Here's how the part is built. I have some questions about the finished solid (model axes, mm). A direction names the side the tool comes from. Round coordinates to 2 decimals unless told otherwise and drop trailing zeros. Order: outer loops, then holes, each group sorted by start corner. A loop starts at its lowest first (then second) coordinate and runs counter-clockwise, first axis right, second up. Notation, with made-up numbers: (22, 35.25) -> (79, 35.25) arc R8 cw to (79, 39.25) -> close; hole circle Ø5 at (-22, 35.25). An arc over 180 degrees is marked (long way). Use a Markdown table: item, result. Add a question column.
(1) I want a section at D-D, the plane z = 1. Give the number of separate pieces and of enclosed holes in the cut face, then the cut area to 3 significant figures.
(2) I want a section at A-A, the plane x = -1.5. Please give me the cut outline in (y, z).
(3) I want a section at C-C, the plane x = -8.5. Please give me the cut outline in (y, z).
(4) If I drill on probe 1 along Y at (x, z) = (0, 1); probe 2 along Y at (x, z) = (-3, 5.5); probe 3 along X at (y, z) = (-3.75, 0.5), over which ranges is the centre line in solid material (lowest first)?
(5) Thinking about a two-plate mould opening in X: for faces 4 (the face through (0, -7.05, 22)), 5 (the face through (-14.42, -4.03, 21.76)), 6 (the face through (6.9, 0, 2)), which applies, pulls with the +X half, pulls with the -X half, needs draft (parallel to the pull), parting line crosses it, or undercut?
(6) On a 3-axis mill with a long thin cutter (end or side, diameter ignored), from which of +Z, -Z, +X, -X, +Y, -Y can I reach the whole of each face in a straight line? I mean faces 1 (the face through (0, 2.8, -1)), 2 (the face through (-14.48, 3.97, 21.76)), 3 (the face through (-12.15, -2, 22)). Say none if no direction works.
(7) I'm going to push flat-ended pins straight in: P1, Ø6, axis at x = -0.5, y = 0, coming from the +Z side; P2, Ø1, axis at x = -13.5, z = 36.5, coming from the -Y side; P3, Ø0.6, axis at x = -13.5, z = 28, coming from the +Y side. Where does each tip first touch, or does it pass through?
from build123d import *

# Parameters (mm, degrees)
F1_DEPTH     = 2
F2_DEPTH     = 5
F3_DEPTH     = 44
F4_DEPTH     = 46.2
F6_T1_DEPTH  = 6.8
F6_T3_DEPTH  = 13.8
F6_T9_DEPTH  = 16.371682988
F6_T15_DEPTH = 9.371682988
F6_T24_DEPTH = 9.371682988
F6_T30_DEPTH = 16.371682988
F6_T39_DEPTH = 16.371682988
F6_T45_DEPTH = 9.371682988
F6_T54_DEPTH = 16.371682988
F6_T60_DEPTH = 9.371682988


# Not quite as in the source:
# - a fillet or chamfer that OpenCascade refuses, or shapes differently, is made with other operations: its cross-section is extruded or revolved along the edge and cut away or added
# - a feature names something its author has since deleted; it is built from what else it names


with BuildPart() as f1:
    # F0 (on Top) → F1 (new body)
    with BuildSketch(Plane.XY):
        with BuildLine():
            Line((10.3671572875, 5.05), (0, 5.05))
            Line((0, 5.05), (0, 4.2))
            Line((0, 4.2), (7.7, 4.2))
            Line((7.7, 4.2), (7.7, -4.2))
            Line((7.7, -4.2), (0, -4.2))
            Line((0, -4.2), (0, -5.05))
            Line((0, -5.05), (10.3671572875, -5.05))
            ThreePointArc((10.3671572875, -5.05), (10.5584990037, -5.0119397663), (10.7207106781, -4.9035533906))
            Line((10.7207106781, -4.9035533906), (12.15, -3.4742640687))
            Line((12.15, -3.4742640687), (12.15, -1.4742640687))
            Line((12.15, -1.4742640687), (14.15, -1.4742640687))
            Line((14.15, -1.4742640687), (15.2707106781, -0.3535533906))
            ThreePointArc((15.2707106781, -0.3535533906), (15.4171572875, 0), (15.2707106781, 0.3535533906))
            Line((15.2707106781, 0.3535533906), (10.7207106781, 4.9035533906))
            ThreePointArc((10.7207106781, 4.9035533906), (10.5584990037, 5.0119397663), (10.3671572875, 5.05))
        make_face()
        Polygon((6.9, 3.4), (0, 3.4), (0, 2.8), (6.3, 2.8), (6.3, -2.8), (0, -2.8), (0, -3.4), (6.9, -3.4), align=None)
        Polygon((7.7, 4.2), (0, 4.2), (0, 3.4), (6.9, 3.4), (6.9, -3.4), (0, -3.4), (0, -4.2), (7.7, -4.2), align=None)
        with BuildLine():
            Line((10.45, 7.05), (0, 7.05))
            Line((0, 7.05), (0, 5.85))
            Line((0, 5.85), (10.3671572875, 5.85))
            ThreePointArc((10.3671572875, 5.85), (10.8646457496, 5.7510433923), (11.2863961031, 5.4692388155))
            Line((11.2863961031, 5.4692388155), (15.8363961031, 0.9192388155))
            ThreePointArc((15.8363961031, 0.9192388155), (16.2171572875, 0), (15.8363961031, -0.9192388155))
            Line((15.8363961031, -0.9192388155), (11.2863961031, -5.4692388155))
            ThreePointArc((11.2863961031, -5.4692388155), (10.8646457496, -5.7510433923), (10.3671572875, -5.85))
            Line((10.3671572875, -5.85), (0, -5.85))
            Line((0, -5.85), (0, -7.05))
            Line((0, -7.05), (10.45, -7.05))
            ThreePointArc((10.45, -7.05), (11.3301718944, -6.8749229248), (12.0763455967, -6.3763455967))
            Line((12.0763455967, -6.3763455967), (16.8263455967, -1.6263455967))
            ThreePointArc((16.8263455967, -1.6263455967), (17.5, 0), (16.8263455967, 1.6263455967))
            Line((16.8263455967, 1.6263455967), (12.0763455967, 6.3763455967))
            ThreePointArc((12.0763455967, 6.3763455967), (11.3301718944, 6.8749229248), (10.45, 7.05))
        make_face()
        with BuildLine():
            Line((10.3671572875, 5.85), (0, 5.85))
            Line((0, 5.85), (0, 5.05))
            Line((0, 5.05), (10.3671572875, 5.05))
            ThreePointArc((10.3671572875, 5.05), (10.5584990037, 5.0119397663), (10.7207106781, 4.9035533906))
            Line((10.7207106781, 4.9035533906), (15.2707106781, 0.3535533906))
            ThreePointArc((15.2707106781, 0.3535533906), (15.4171572875, 0), (15.2707106781, -0.3535533906))
            Line((15.2707106781, -0.3535533906), (14.15, -1.4742640687))
            Line((14.15, -1.4742640687), (12.15, -1.4742640687))
            Line((12.15, -1.4742640687), (12.15, -3.4742640687))
            Line((12.15, -3.4742640687), (10.7207106781, -4.9035533906))
            ThreePointArc((10.7207106781, -4.9035533906), (10.5584990037, -5.0119397663), (10.3671572875, -5.05))
            Line((10.3671572875, -5.05), (0, -5.05))
            Line((0, -5.05), (0, -5.85))
            Line((0, -5.85), (10.3671572875, -5.85))
            ThreePointArc((10.3671572875, -5.85), (10.8646457496, -5.7510433923), (11.2863961031, -5.4692388155))
            Line((11.2863961031, -5.4692388155), (15.8363961031, -0.9192388155))
            ThreePointArc((15.8363961031, -0.9192388155), (16.2171572875, 0), (15.8363961031, 0.9192388155))
            Line((15.8363961031, 0.9192388155), (11.2863961031, 5.4692388155))
            ThreePointArc((11.2863961031, 5.4692388155), (10.8646457496, 5.7510433923), (10.3671572875, 5.85))
        make_face()
    extrude(amount=-F1_DEPTH)

    # F0 (on Top) → F2 (join)
    with BuildSketch(Plane.XY):
        Polygon((7.7, 4.2), (0, 4.2), (0, 3.4), (6.9, 3.4), (6.9, -3.4), (0, -3.4), (0, -4.2), (7.7, -4.2), align=None)
    extrude(amount=F2_DEPTH)

    # F0 (on Top) → F3 (join)
    with BuildSketch(Plane.XY):
        with BuildLine():
            Line((10.3671572875, 5.85), (0, 5.85))
            Line((0, 5.85), (0, 5.05))
            Line((0, 5.05), (10.3671572875, 5.05))
            ThreePointArc((10.3671572875, 5.05), (10.5584990037, 5.0119397663), (10.7207106781, 4.9035533906))
            Line((10.7207106781, 4.9035533906), (15.2707106781, 0.3535533906))
            ThreePointArc((15.2707106781, 0.3535533906), (15.4171572875, 0), (15.2707106781, -0.3535533906))
            Line((15.2707106781, -0.3535533906), (14.15, -1.4742640687))
            Line((14.15, -1.4742640687), (12.15, -1.4742640687))
            Line((12.15, -1.4742640687), (12.15, -3.4742640687))
            Line((12.15, -3.4742640687), (10.7207106781, -4.9035533906))
            ThreePointArc((10.7207106781, -4.9035533906), (10.5584990037, -5.0119397663), (10.3671572875, -5.05))
            Line((10.3671572875, -5.05), (0, -5.05))
            Line((0, -5.05), (0, -5.85))
            Line((0, -5.85), (10.3671572875, -5.85))
            ThreePointArc((10.3671572875, -5.85), (10.8646457496, -5.7510433923), (11.2863961031, -5.4692388155))
            Line((11.2863961031, -5.4692388155), (15.8363961031, -0.9192388155))
            ThreePointArc((15.8363961031, -0.9192388155), (16.2171572875, 0), (15.8363961031, 0.9192388155))
            Line((15.8363961031, 0.9192388155), (11.2863961031, 5.4692388155))
            ThreePointArc((11.2863961031, 5.4692388155), (10.8646457496, 5.7510433923), (10.3671572875, 5.85))
        make_face()
    extrude(amount=F3_DEPTH)

    # F0 (on Top) → F4 (join)
    with BuildSketch(Plane.XY):
        with BuildLine():
            Line((10.45, 7.05), (0, 7.05))
            Line((0, 7.05), (0, 5.85))
            Line((0, 5.85), (10.3671572875, 5.85))
            ThreePointArc((10.3671572875, 5.85), (10.8646457496, 5.7510433923), (11.2863961031, 5.4692388155))
            Line((11.2863961031, 5.4692388155), (15.8363961031, 0.9192388155))
            ThreePointArc((15.8363961031, 0.9192388155), (16.2171572875, 0), (15.8363961031, -0.9192388155))
            Line((15.8363961031, -0.9192388155), (11.2863961031, -5.4692388155))
            ThreePointArc((11.2863961031, -5.4692388155), (10.8646457496, -5.7510433923), (10.3671572875, -5.85))
            Line((10.3671572875, -5.85), (0, -5.85))
            Line((0, -5.85), (0, -7.05))
            Line((0, -7.05), (10.45, -7.05))
            ThreePointArc((10.45, -7.05), (11.3301718944, -6.8749229248), (12.0763455967, -6.3763455967))
            Line((12.0763455967, -6.3763455967), (16.8263455967, -1.6263455967))
            ThreePointArc((16.8263455967, -1.6263455967), (17.5, 0), (16.8263455967, 1.6263455967))
            Line((16.8263455967, 1.6263455967), (12.0763455967, 6.3763455967))
            ThreePointArc((12.0763455967, 6.3763455967), (11.3301718944, 6.8749229248), (10.45, 7.05))
        make_face()
    extrude(amount=F4_DEPTH)

    # F5: F1 across face


with BuildPart() as f1_1:
    add(f1.part)
    add(f1.part.mirror(Plane(origin=(0, 5.8802646888, 19.9395384914), x_dir=(0, -1, 0), z_dir=(-1, 0, 0))))

    # F6: chamfer of 1 on 4 edges, made by hand

    # F6_s2 → F6_t1 (cut)
    with BuildSketch(Plane.XZ.offset(-3.4)):
        Polygon((7.9, 5), (6.9, 4), (6.9, 5), align=None)
        Polygon((-7.9, 5), (-6.9, 4), (-6.9, 5), align=None)
    extrude(amount=F6_T1_DEPTH, mode=Mode.SUBTRACT)

    # F6_s4 → F6_t3 (cut)
    with BuildSketch(Plane.YZ.offset(-6.9)):
        Polygon((4.4, 5), (3.4, 4), (3.4, 5), align=None)
        Polygon((-4.4, 5), (-3.4, 4), (-3.4, 5), align=None)
    extrude(amount=F6_T3_DEPTH, mode=Mode.SUBTRACT)


with BuildPart() as f6_tool7:
    # F6_s8 → F6_t9 (new body)
    with BuildSketch(Plane.YZ.offset(9.471682988)):
        Polygon((4.4, 5), (3.4, 4), (3.4, 5), align=None)
    extrude(amount=-F6_T9_DEPTH)

    split(bisect_by=Plane.YZ.offset(7.7), keep=Keep.BOTTOM)

    split(bisect_by=Plane.YZ.offset(6.9), keep=Keep.TOP)

    split(bisect_by=Plane.XZ.offset(-4.2), keep=Keep.TOP)


with BuildPart() as f6_tool13:
    # F6_s14 → F6_t15 (new body)
    with BuildSketch(Plane.XZ.offset(-5.971682988)):
        Polygon((7.9, 5), (6.9, 4), (6.9, 5), align=None)
    extrude(amount=F6_T15_DEPTH)

    split(bisect_by=Plane.YZ.offset(7.7), keep=Keep.BOTTOM)

    split(bisect_by=Plane.XZ.offset(-3.4), keep=Keep.BOTTOM)

    split(bisect_by=Plane.XZ.offset(-4.2), keep=Keep.TOP)


with BuildPart() as f6_tool7_1:
    add(f6_tool7.part)

    # F6_t19: intersect F6_tool13
    add(f6_tool13.part, mode=Mode.INTERSECT)


with BuildPart() as f1_2:
    add(f1_1.part)

    # F6_t5: cut F6_tool7
    add(f6_tool7_1.part, mode=Mode.SUBTRACT)


with BuildPart() as f6_tool22:
    # F6_s23 → F6_t24 (new body)
    with BuildSketch(Plane.XZ.offset(-3.4)):
        Polygon((7.9, 5), (6.9, 4), (6.9, 5), align=None)
    extrude(amount=F6_T24_DEPTH)

    split(bisect_by=Plane.YZ.offset(7.7), keep=Keep.BOTTOM)

    split(bisect_by=Plane.XZ.offset(3.4), keep=Keep.TOP)

    split(bisect_by=Plane.XZ.offset(4.2), keep=Keep.BOTTOM)


with BuildPart() as f6_tool28:
    # F6_s29 → F6_t30 (new body)
    with BuildSketch(Plane.YZ.offset(-6.9)):
        Polygon((-4.4, 5), (-3.4, 4), (-3.4, 5), align=None)
    extrude(amount=F6_T30_DEPTH)

    split(bisect_by=Plane.YZ.offset(7.7), keep=Keep.BOTTOM)

    split(bisect_by=Plane.YZ.offset(6.9), keep=Keep.TOP)

    split(bisect_by=Plane.XZ.offset(4.2), keep=Keep.BOTTOM)


with BuildPart() as f6_tool22_1:
    add(f6_tool22.part)

    # F6_t34: intersect F6_tool28
    add(f6_tool28.part, mode=Mode.INTERSECT)


with BuildPart() as f1_3:
    add(f1_2.part)

    # F6_t20: cut F6_tool22
    add(f6_tool22_1.part, mode=Mode.SUBTRACT)


with BuildPart() as f6_tool37:
    # F6_s38 → F6_t39 (new body)
    with BuildSketch(Plane.YZ.offset(6.9)):
        Polygon((4.4, 5), (3.4, 4), (3.4, 5), align=None)
    extrude(amount=-F6_T39_DEPTH)

    split(bisect_by=Plane.YZ.offset(-6.9), keep=Keep.BOTTOM)

    split(bisect_by=Plane.XZ.offset(-4.2), keep=Keep.TOP)

    split(bisect_by=Plane.YZ.offset(-7.7), keep=Keep.TOP)


with BuildPart() as f6_tool43:
    # F6_s44 → F6_t45 (new body)
    with BuildSketch(Plane.XZ.offset(-5.971682988)):
        Polygon((-7.9, 5), (-6.9, 4), (-6.9, 5), align=None)
    extrude(amount=F6_T45_DEPTH)

    split(bisect_by=Plane.XZ.offset(-3.4), keep=Keep.BOTTOM)

    split(bisect_by=Plane.XZ.offset(-4.2), keep=Keep.TOP)

    split(bisect_by=Plane.YZ.offset(-7.7), keep=Keep.TOP)


with BuildPart() as f6_tool37_1:
    add(f6_tool37.part)

    # F6_t49: intersect F6_tool43
    add(f6_tool43.part, mode=Mode.INTERSECT)


with BuildPart() as f1_4:
    add(f1_3.part)

    # F6_t35: cut F6_tool37
    add(f6_tool37_1.part, mode=Mode.SUBTRACT)


with BuildPart() as f6_tool52:
    # F6_s53 → F6_t54 (new body)
    with BuildSketch(Plane.YZ.offset(-9.471682988)):
        Polygon((-4.4, 5), (-3.4, 4), (-3.4, 5), align=None)
    extrude(amount=F6_T54_DEPTH)

    split(bisect_by=Plane.YZ.offset(-6.9), keep=Keep.BOTTOM)

    split(bisect_by=Plane.YZ.offset(-7.7), keep=Keep.TOP)

    split(bisect_by=Plane.XZ.offset(4.2), keep=Keep.BOTTOM)


with BuildPart() as f6_tool58:
    # F6_s59 → F6_t60 (new body)
    with BuildSketch(Plane.XZ.offset(-3.4)):
        Polygon((-7.9, 5), (-6.9, 4), (-6.9, 5), align=None)
    extrude(amount=F6_T60_DEPTH)

    split(bisect_by=Plane.XZ.offset(3.4), keep=Keep.TOP)

    split(bisect_by=Plane.YZ.offset(-7.7), keep=Keep.TOP)

    split(bisect_by=Plane.XZ.offset(4.2), keep=Keep.BOTTOM)


with BuildPart() as f6_tool52_1:
    add(f6_tool52.part)

    # F6_t64: intersect F6_tool58
    add(f6_tool58.part, mode=Mode.INTERSECT)


with BuildPart() as f1_5:
    add(f1_4.part)

    # F6_t50: cut F6_tool52
    add(f6_tool52_1.part, mode=Mode.SUBTRACT)


solid = f1_5.part
Taken from the geometry:
| question | item | result |
|---|---|---|
| 1 | separate pieces | 2 |
| 1 | enclosed holes | 2 |
| 1 | area | 193 mm2 |
| 2 | outline | (-7.05, -2) -> (-2.8, -2) -> (-2.8, 0) -> (-3.4, 0) -> (-3.4, 4) -> (-4.2, 4.8) -> (-4.2, 0) -> (-5.05, 0) -> (-5.05, 44) -> (-5.85, 44) -> (-5.85, 46.2) -> (-7.05, 46.2) -> close; (2.8, -2) -> (7.05, -2) -> (7.05, 46.2) -> (5.85, 46.2) -> (5.85, 44) -> (5.05, 44) -> (5.05, 0) -> (4.2, 0) -> (4.2, 4.8) -> (3.4, 4) -> (3.4, 0) -> (2.8, 0) -> close |
| 3 | outline | (-7.05, -2) -> (7.05, -2) -> (7.05, 46.2) -> (5.85, 46.2) -> (5.85, 44) -> (5.05, 44) -> (5.05, 0) -> (-5.05, 0) -> (-5.05, 44) -> (-5.85, 44) -> (-5.85, 46.2) -> (-7.05, 46.2) -> close |
| 4 | probe 1 | y = -7.05 to -5.05, -4.2 to -3.4, 3.4 to 4.2, 5.05 to 7.05 |
| 4 | probe 2 | y = -7.05 to -5.05, 5.05 to 7.05 |
| 4 | probe 3 | x = -14.7 to -11.87, -7.7 to 7.7, 11.87 to 14.7 |
| 5 | face 4 | needs draft |
| 5 | face 5 | pulls with the -X half |
| 5 | face 6 | undercut |
| 6 | face 1 | +Z, -Z |
| 6 | face 2 | +Z, -Z, -X, +Y |
| 6 | face 3 | +Z |
| 7 | P1 | stops at z = 0 |
| 7 | P2 | stops at y = -5.45 |
| 7 | P3 | stops at y = 5.25 |
